The listing builds one solid part. Answer for the finished solid, in the listing's coordinates (mm). Give positions to 0.01 mm unless a question says otherwise; leave off trailing zeros. Write each loop counter-clockwise with the first axis right and the second up, starting at its lowest first coordinate (ties: lowest second). Pieces come first, ordered by that corner, then holes. Notation, with made-up numbers: M 30,74 L 58,74 A20 ccw 58,87 Z; hole C 18,21.5 d5. An arc over 180 degrees is marked long. Answer as a JSON object with one key per item and string values.
```python
from build123d import *

# Parameters (mm, degrees)
F0_W     = 101.6
F0_H     = 101.6
F1_DEPTH = 50.8
F2_R     = 31.75
F3_DEPTH = 101.601
F4_R     = 6.517177
F5_DEPTH = 101.601


with BuildPart() as f1:
    # F0 (on Front) → F1 (new body, symmetric)
    with BuildSketch(Plane.XZ):
        Rectangle(F0_W, F0_H)
    extrude(amount=F1_DEPTH, both=True)

    # F2 (on face) → F3 (cut, through all)
    with BuildSketch(Plane.XY.offset(50.8)):
        Circle(F2_R)
    extrude(amount=-F3_DEPTH, mode=Mode.SUBTRACT)

    # F4 (on face) → F5 (cut, through all)
    with BuildSketch(Plane.XY.offset(50.8)):
        with Locations((-37.914988, -30.449271)):
            Circle(F4_R)
    extrude(amount=-F5_DEPTH, mode=Mode.SUBTRACT)


solid = f1.part
```
1. A cutting plane is placed at A-A, the plane x = 0. Give the vertices of the cut face in (y, z).
Verdict:
{"outline": "M -50.8,-50.8 L -31.75,-50.8 L -31.75,50.8 L -50.8,50.8 Z; M 31.75,-50.8 L 50.8,-50.8 L 50.8,50.8 L 31.75,50.8 Z"}
2. The mould has two halves that part along X. Classify faces 1 (the flat face through (21.9, -23.3, -50.8)), 2 (the cylindrical face through (-31.7, -28.49, 0.71)), 3 (the cylindrical face through (-6.883, -30.995, 0.711)), 4 (the flat face through (50.8, -1, -1)): released by +X, released by -X, zero draft, split by the parting line, or undercut.
Verdict:
{"face 1": "zero draft", "face 2": "undercut", "face 3": "undercut", "face 4": "released by +X"}
3. Consider line 1 along Y through (x, z) = (0, 30); line 2 along X through (y, z) = (-27.5, 46.5); line 3 along X through (y, z) = (-1, 35). Determine where each line is inside the solid, lowest interval first.
Verdict:
{"line 1": "y = -50.8 to -31.75, 31.75 to 50.8", "line 2": "x = -50.8 to -43.73, -32.1 to -15.87, 15.87 to 50.8", "line 3": "x = -50.8 to -31.73, 31.73 to 50.8"}
4. A cutting plane is placed at B-B, the plane y = -5.5. Give the vertices of the cut face in (x, z), plus the area to 3 significant figures.
Verdict:
{"outline": "M -50.8,-50.8 L -31.27,-50.8 L -31.27,50.8 L -50.8,50.8 Z; M 31.27,-50.8 L 50.8,-50.8 L 50.8,50.8 L 31.27,50.8 Z", "area": "3,970 mm2"}
5. A cutting plane is placed at C-C, the plane z = -28. Give the vertices of the cut face in (x, y).
Verdict:
{"outline": "M -50.8,-50.8 L 50.8,-50.8 L 50.8,50.8 L -50.8,50.8 Z; hole C -37.91,-30.45 d13.03; hole C 0,0 d63.5"}
